Check sheet for the drawn part. Datum: minimum x, y, z corner. Units: mm. Round coordinates to 2 decimals unless told otherwise and drop trailing zeros. Write each loop counter-clockwise with the first axis right and the second up, starting at its lowest first coordinate (ties: lowest second). Pieces come first, ordered by that corner, then holes. Notation, with made-up numbers: (88.5, -29.5) - (146.5, -29.5) arc R37 cw to (146.5, 8.5) - close; hole circle Ø9 at (-35, 48.5). An arc over 180 degrees is marked (long way). Write each question's results on one line, items separated by ' | '.
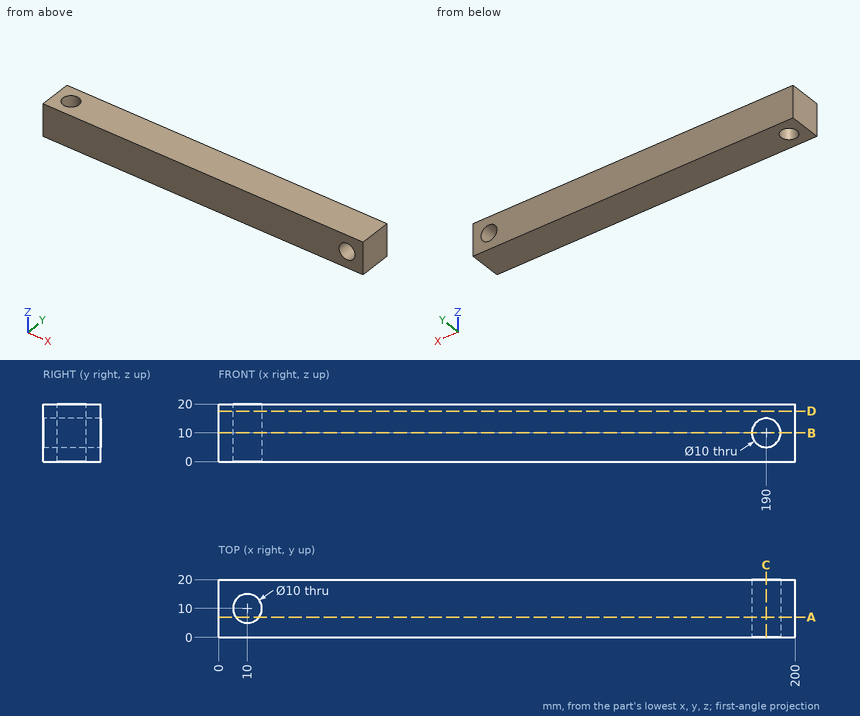
(1) Section check C-C (x = 190). Record the cut outline in (y, z), plus the area to 3 significant figures.
Answer:
outline: (0, 0) - (20, 0) - (20, 5) - (0, 5) - close; (0, 15) - (20, 15) - (20, 20) - (0, 20) - close | area: 200 mm2
(2) Section check D-D (z = 17.5). Record the cut outline in (x, y).
Answer:
outline: (0, 0) - (200, 0) - (200, 20) - (0, 20) - close; hole circle Ø10 at (10, 10)
(3) Section check A-A (y = 7). Record the cut outline in (x, z), plus the area to 3 significant figures.
Answer:
outline: (0, 0) - (6, 0) - (6, 20) - (0, 20) - close; (14, 0) - (200, 0) - (200, 20) - (14, 20) - close; hole circle Ø10 at (190, 10) | area: 3,760 mm2
(4) Section check B-B (z = 10). Record the cut outline in (x, y).
Answer:
outline: (0, 0) - (185, 0) - (185, 20) - (0, 20) - close; (195, 0) - (200, 0) - (200, 20) - (195, 20) - close; hole circle Ø10 at (10, 10)
(5) Thickness scan on L1, parallel to Z at x = 190, y = 11.5; L2, parallel to X at y = 8, z = 1.75; L3, parallel to X at y = 16, z = 6.5. Record the ranges inside material, lowest first.
Answer:
L1: 0 to 5, 15 to 20 | L2: 0 to 5.42, 14.58 to 200 | L3: 0 to 186.43, 193.57 to 200
(6) Go/stop test with a flat-tipped pin: pin 1 Ø9 at (x, z) = (190, 10) entering from -Y. Record where the tip stops, or that it passes through.
Answer:
pin 1: through
